from build123d import *
from build123d.topology import SkipClean

# Parameters (mm, degrees)
SKETCH2_W                = 32
SKETCH2_H                = 30
BOSS_EXTRUDE1_DEPTH      = 2.922658801
BOSS_EXTRUDE2_DEPTH      = 25
BOSS_EXTRUDE2_DEPTH_BACK = 2.922659
SKETCH3_W                = 8
SKETCH3_H                = 30
CUT_EXTRUDE1_DEPTH       = 58.521082001
CUT_EXTRUDE1_DEPTH_BACK  = 58.521082001
SKETCH4_R                = 8
M3X0_5_TAPPED_HOLE1_D    = 2.5
SKETCH7_R                = 2.5
CUT_EXTRUDE2_DEPTH       = 38.762415177
SKETCH8_W                = 30
SKETCH8_H                = 18.9613294
CUT_EXTRUDE3_DEPTH       = 58.521082001
M3_CLEARANCE_HOLE1_D     = 3.2
CHAMFER1_SIZE            = 0.5
SKETCH13_R               = 3
CUT_EXTRUDE4_DEPTH       = 4


with BuildPart() as part:
    # Sketch2 → Boss-Extrude1 (new body)
    with BuildSketch(Plane(origin=(0, 0, 0), x_dir=(1, 0, 0), z_dir=(0, 1, 0))):
        Rectangle(SKETCH2_W, SKETCH2_H)
    extrude(amount=BOSS_EXTRUDE1_DEPTH)

    # Sketch3 → Boss-Extrude2 (add, two sides: drawn at the far end of the back side and taken through both)
    with BuildSketch(Plane(origin=(0, 2.922658801, 0), x_dir=(1, 0, 0), z_dir=(0, 1, 0)).offset(-BOSS_EXTRUDE2_DEPTH_BACK)):
        with Locations((-20, 0)):
            Rectangle(SKETCH3_W, SKETCH3_H)
        with Locations((20, 0)):
            Rectangle(SKETCH3_W, SKETCH3_H)
    extrude(amount=BOSS_EXTRUDE2_DEPTH + BOSS_EXTRUDE2_DEPTH_BACK)

    # Sketch4 → Cut-Extrude1 (cut, two sides: drawn at the far end of the back side and taken through both)
    with BuildSketch(Plane(origin=(24, 0, 0), x_dir=(0, 0, -1), z_dir=(1, 0, 0)).offset(-CUT_EXTRUDE1_DEPTH_BACK)):
        with Locations((0, 13.961329401)):
            Circle(SKETCH4_R)
    extrude(amount=CUT_EXTRUDE1_DEPTH + CUT_EXTRUDE1_DEPTH_BACK, mode=Mode.SUBTRACT)

    # M3x0.5 Tapped Hole1 (through all)
    with Locations(Plane(origin=(0, 2.922658801, 0), x_dir=(1, 0, 0), z_dir=(0, 1, 0))):
        with Locations((12, 0), (0, 0), (-12, 0)):
            Hole(M3X0_5_TAPPED_HOLE1_D / 2)

    # Sketch7 → Cut-Extrude2 (cut, through all)
    with BuildSketch(Plane(origin=(0, 2.922658801, 0), x_dir=(1, 0, 0), z_dir=(0, 1, 0))):
        with Locations(Location((-11, 7.5, 0), (0, 0, 270))):
            Circle(SKETCH7_R)
        with Locations(Location((-11, -7.5, 0), (0, 0, 270))):
            Circle(SKETCH7_R)
        with Locations(Location((11, -7.5, 0), (0, 0, 270))):
            Circle(SKETCH7_R)
        with Locations(Location((11, 7.5, 0), (0, 0, 270))):
            Circle(SKETCH7_R)
        with BuildLine():
            Line((-3, 11.5), (3, 11.5))
            ThreePointArc((3, 11.5), (7, 7.5), (3, 3.5))
            Line((3, 3.5), (-3, 3.5))
            ThreePointArc((-3, 3.5), (-7, 7.5), (-3, 11.5))
        make_face()
        with BuildLine():
            Line((-3, -3.5), (3, -3.5))
            ThreePointArc((3, -3.5), (7, -7.5), (3, -11.5))
            Line((3, -11.5), (-3, -11.5))
            ThreePointArc((-3, -11.5), (-7, -7.5), (-3, -3.5))
        make_face()
    extrude(amount=-CUT_EXTRUDE2_DEPTH, mode=Mode.SUBTRACT)

    # Sketch8 → Cut-Extrude3 (cut, through all)
    with BuildSketch(Plane(origin=(24, 0, 0), x_dir=(0, 0, -1), z_dir=(1, 0, 0))):
        with Locations((0, 23.441994101)):
            Rectangle(SKETCH8_W, SKETCH8_H)
    extrude(amount=-CUT_EXTRUDE3_DEPTH, mode=Mode.SUBTRACT)

    # M3 Clearance Hole1 (through all)
    with Locations(Plane(origin=(0, 0, 0), x_dir=(-1, 0, 0), z_dir=(0, -1, 0))):
        with Locations((-20, 11.49), (20, -11.49), (-20, -11.49), (20, 11.49)):
            Hole(M3_CLEARANCE_HOLE1_D / 2)

    # Chamfer1
    chamfer1_edges = [part.edges().sort_by_distance(p)[0] for p in [
        (-16, 5.961329401, 0),
        (-24, 5.961329401, 0),
        (16, 5.961329401, 0),
        (24, 5.961329401, 0),
        (-16, 8.441994101, -15),
        (-16, 8.441994101, 15),
        (-24, 6.980664601, 15),
        (-24, 6.980664601, -15),
        (-24, -1.99e-07, 0),
        (0, 2.922658801, -15),
        (16, 8.441994101, 15),
        (16, 8.441994101, -15),
        (24, 6.980664601, -15),
        (24, 6.980664601, 15),
        (24, -1.99e-07, 0),
        (0, 0, -15),
        (0, 0, 15),
        (0, 2.922658801, 15),
    ]]
    chamfer(chamfer1_edges, length=CHAMFER1_SIZE)

    # Sketch13 → Cut-Extrude4 (cut)
    with SkipClean():  # the faces are left unmerged after this step: merging them gives an invalid solid
        with BuildSketch(Plane.XZ):
            with Locations(Location((20, -11.49, 0), (0, 0, 270))):
                Circle(SKETCH13_R)
            with Locations(Location((-20, -11.49, 0), (0, 0, 270))):
                Circle(SKETCH13_R)
            with Locations(Location((-20, 11.49, 0), (0, 0, 270))):
                Circle(SKETCH13_R)
            with Locations(Location((20, 11.49, 0), (0, 0, 270))):
                Circle(SKETCH13_R)
        extrude(amount=-CUT_EXTRUDE4_DEPTH, mode=Mode.SUBTRACT)


solid = part.part
Source: CAD feature listing. Evaluate the final solid. Frame: model axes, mm. A direction names the side the tool comes from. Round coordinates to 2 decimals unless told otherwise and drop trailing zeros. Write each loop counter-clockwise with the first axis right and the second up, starting at its lowest first coordinate (ties: lowest second). Pieces come first, ordered by that corner, then holes. Notation, with made-up numbers: (33, 12.5) - (48, 12.5) arc R16 ccw to (48, 34.5) - close; hole circle Ø7 at (32, 75). An arc over 180 degrees is marked (long way). Use CSV: the item, a comma, the result in double quotes. Start each with the question number.
(1) Mould query, pull axis X, two halves, no side actions, for faces 1 (the face through (-24, 4, 0)), 2 (the face through (19.951, 5.963, 0.176)), 3 (the face through (0, 1, 11.5)). Classes: pulls with the +X half, pulls with the -X half, needs draft (parallel to the pull), parting line crosses it, or undercut.
(2) Cut plane C-C, the plane x = 0. Return loops of the section in (y, z), and give its area (3 significant figures).
(3) Cut plane B-B, the plane x = -20. Give the number of separate pieces and of enclosed holes in the cut face, and give its area (3 significant figures).
(4) Set-up query: faces 4 (the face through (-22.662, 1.972, 10.106)), 5 (the face through (-7, 1.5, 7.6)), 6 (the face through (-16, 5, 0)). Return all of +Z, -Z, +X, -X, +Y, -Y with unobstructed straight access to the full face (end or side cutting, diameter ignored); none if empty.
(5) Cut plane A-A, the plane z = 0. Return loops of the section in (x, y).
(6) First-contact query: pin 1 Ø8 at (y, z) = (7, 0.5) entering from +X; pin 2 Ø6 at (y, z) = (11.5, -4) entering from +X; pin 3 Ø3.5 at (x, z) = (-20, -11.49) entering from -Y; pin 4 Ø4 at (x, z) = (5.5, -5.5) entering from +Y. Flat tips, straight axial feed; report the tip coordinate or a pass-through.
(7) Material intervals for probe 1 along X at (y, z) = (2, 7.5); probe 2 along X at (y, z) = (6.5, 11.49); probe 3 along Z at (x, y) = (13, 2.25), sorted ascending. Write a range as [from, to].
Geometry says:
1,face 1,"pulls with the -X half"
1,face 2,"needs draft"
1,face 3,"undercut"
2,outline,"(0, -14.5) - (0.5, -15) - (2.42, -15) - (2.92, -14.5) - (2.92, -11.5) - (0, -11.5) - close; (0, -3.5) - (2.92, -3.5) - (2.92, -1.25) - (0, -1.25) - close; (0, 1.25) - (2.92, 1.25) - (2.92, 3.5) - (0, 3.5) - close; (0, 11.5) - (2.92, 11.5) - (2.92, 14.5) - (2.42, 15) - (0.5, 15) - (0, 14.5) - close"
2,area,"33.1 mm²"
3,separate pieces,"3"
3,enclosed holes,"0"
3,area,"206 mm²"
4,face 4,"-Y"
4,face 5,"+Y, -Y"
4,face 6,"+Z, -Z, +Y"
5,outline,"(-24, 0.5) - (-23.5, 0) - (-13.25, 0) - (-13.25, 2.92) - (-16, 2.92) - (-16, 5.46) - (-16.5, 5.96) - (-23.5, 5.96) - (-24, 5.46) - close; (-10.75, 0) - (-1.25, 0) - (-1.25, 2.92) - (-10.75, 2.92) - close; (1.25, 0) - (10.75, 0) - (10.75, 2.92) - (1.25, 2.92) - close; (13.25, 0) - (23.5, 0) - (24, 0.5) - (24, 5.46) - (23.5, 5.96) - (16.5, 5.96) - (16, 5.46) - (16, 2.92) - (13.25, 2.92) - close"
6,pin 1,"x = 24"
6,pin 2,"through"
6,pin 3,"y = 4"
6,pin 4,"y = 2.92"
7,probe 1,"[-24, -13.5], [-8.5, -7], [7, 8.5], [13.5, 24]"
7,probe 2,"[-24, -21.6], [-18.4, -16], [16, 18.4], [21.6, 24]"
7,probe 3,"[-15, -9], [-6, -0.75], [0.75, 6], [9, 15]"
